from build123d import *

# Parameters (mm, degrees)
SKETCH1_R            = 28.1
SKETCH1_R_2          = 21.1
BOSS_EXTRUDE1_DEPTH  = 4.5
SKETCH2_R            = 28.1
SKETCH2_R_2          = 18.6
BOSS_EXTRUDE2_DEPTH  = 3
M3_CLEARANCE_HOLE1_D = 3.2
SKETCH6_R            = 3
CUT_EXTRUDE1_DEPTH   = 2
BOSS_EXTRUDE3_DEPTH  = 10
SKETCH8_R            = 2.125
CUT_EXTRUDE2_DEPTH   = 15
SKETCH9_W            = 6.5
SKETCH9_H            = 10
CUT_EXTRUDE3_DEPTH   = 7
CIRPATTERN1_COUNT    = 6
CIRPATTERN2_COUNT    = 2


with BuildPart() as part:
    # Sketch1 → Boss-Extrude1 (new body)
    with BuildSketch(Plane.XY):
        Circle(SKETCH1_R)
        Circle(SKETCH1_R_2, mode=Mode.SUBTRACT)
    extrude(amount=BOSS_EXTRUDE1_DEPTH)

    # Sketch2 → Boss-Extrude2 (add)
    with BuildSketch(Plane.XY.offset(4.5)):
        Circle(SKETCH2_R)
        Circle(SKETCH2_R_2, mode=Mode.SUBTRACT)
    extrude(amount=BOSS_EXTRUDE2_DEPTH)

    # M3 Clearance Hole1 (through all)
    with Locations(Plane(origin=(0, 0, 0), x_dir=(-1, 0, 0), z_dir=(0, 0, -1))):
        with Locations((0, 24.6)):
            m3_clearance_hole1 = Hole(M3_CLEARANCE_HOLE1_D / 2)

    # Sketch6 → Cut-Extrude1 (cut)
    with BuildSketch(Plane.XY.offset(7.5)):
        with Locations((0, 24.6)):
            Circle(SKETCH6_R)
    cut_extrude1 = extrude(amount=-CUT_EXTRUDE1_DEPTH, mode=Mode.SUBTRACT)

    # Sketch7 → Boss-Extrude3 (add)
    with BuildSketch(Plane.XY.offset(7.5)):
        Polygon((-6.504809472, 26.266660498), (-19.495190528, 18.766660498), (-15.995190528, 12.704482672), (-3.004809472, 20.204482672), align=None)
    boss_extrude3 = extrude(amount=BOSS_EXTRUDE3_DEPTH)

    # Sketch8 → Cut-Extrude2 (cut)
    with BuildSketch(Plane(origin=(-6.495190528, -3.75, 0), x_dir=(0, 0, 1), z_dir=(-0.866025404, -0.5, 0))):
        with Locations((14, 22.5)):
            Circle(SKETCH8_R)
    cut_extrude2 = extrude(amount=-CUT_EXTRUDE2_DEPTH, mode=Mode.SUBTRACT)

    # Sketch9 → Cut-Extrude3 (cut)
    with BuildSketch(Plane(origin=(-13, 22.516660498, 0), x_dir=(0.866025404, 0.5, 0), z_dir=(-0.5, 0.866025404, 0))):
        with Locations((0, -12.5)):
            Rectangle(SKETCH9_W, SKETCH9_H)
    cut_extrude3 = extrude(amount=-CUT_EXTRUDE3_DEPTH, mode=Mode.SUBTRACT)

    # CirPattern1: M3 Clearance Hole1, Cut-Extrude1 ×6 about axis
    cirpattern1_axis = Axis((0, 0, 0), (0, 0, 1))
    for i in range(1, CIRPATTERN1_COUNT):
        add(m3_clearance_hole1.rotate(cirpattern1_axis, i * 360 / CIRPATTERN1_COUNT), mode=Mode.SUBTRACT)
        add(cut_extrude1.rotate(cirpattern1_axis, i * 360 / CIRPATTERN1_COUNT), mode=Mode.SUBTRACT)

    # CirPattern2: Boss-Extrude3, Cut-Extrude2, Cut-Extrude3 ×2 about axis
    cirpattern2_axis = Axis((0, 0, 0), (0, 0, 1))
    for i in range(1, CIRPATTERN2_COUNT):
        add(boss_extrude3.rotate(cirpattern2_axis, i * 360 / CIRPATTERN2_COUNT))
        add(cut_extrude2.rotate(cirpattern2_axis, i * 360 / CIRPATTERN2_COUNT), mode=Mode.SUBTRACT)
        add(cut_extrude3.rotate(cirpattern2_axis, i * 360 / CIRPATTERN2_COUNT), mode=Mode.SUBTRACT)


solid = part.part
Can you work these out from the model? Positions are in its coordinate system, mm. A direction names the side the tool comes from. Give positions to 0.01 mm unless a question says otherwise; leave off trailing zeros. Write each loop counter-clockwise with the first axis right and the second up, starting at its lowest first coordinate (ties: lowest second). Pieces come first, ordered by that corner, then holes. Notation, with made-up numbers: M 5,44.25 L 38,44.25 A14 ccw 38,52.25 Z; hole C 62.25,-19.75 d3. An arc over 180 degrees is marked long. Answer in a Markdown table with one row per item. Add a question column.
Item 1: On a 3-axis mill with a long thin cutter (end or side, diameter ignored), from which of +Z, -Z, +X, -X, +Y, -Y can I reach the whole of each face in a straight line? I mean faces 5 (the cylindrical face through (-0.65, 21.67, 6.51)), 6 (the flat face through (17.77, -15.78, 11.32)), 7 (the flat face through (4.73, -23.19, 11.32)), 8 (the flat face through (14.089, -17.903, 11.459)). Say none if no direction works.
Item 2: For pin 1 Ø2 at (x, z) = (7, 9.5) entering from +Y; pin 2 Ø6.5 at (x, y) = (0, 26) entering from +Z; pin 3 Ø8 at (x, z) = (-18, 6) entering from -Y, each with a flat end and sliding along its axis, tell me the tip position at first contact or that it passes through.
Item 3: Imagine slicing it at B-B, the plane x = 0. Write out the boundary of the cut face in (y, z), plus the area to 3 significant figures.
Item 4: Imagine slicing it at D-D, the plane z = 15.25. State how many separate pieces and enclosed holes the cut face has, plus the area to 3 significant figures.
Item 5: We'd pull the mould along Y, two halves only. Please class faces 1 (the cylindrical face through (-6.092, -27.432, 3.698)), 2 (the cylindrical face through (6.668, -22.239, 11.877)), 3 (the flat face through (-17.629, 19.844, 12.43)), 4 (the flat face through (-17.77, 15.78, 11.32)): released by +Y, released by -Y, zero draft, split by the parting line, or undercut.
Item 6: Imagine slicing it at C-C, the plane y = 0. Write out the boundary of the cut face in (x, z).
Item 7: Imagine slicing it at A-A, the plane z = 9.5. Write out the boundary of the cut face in (x, y).
Item 8: Please list where these lines run through material, in increasing order: L1, parallel to Y at x = 0, z = 5.2; L2, parallel to Y at x = 0, z = 6.65; L3, parallel to Z at x = 17.5, y = 20.5.
Evaluation:
| question | item | result |
|---|---|---|
| 1 | face 5 | +Z |
| 1 | face 6 | +Z, +X, +Y |
| 1 | face 7 | +Z, -X, -Y |
| 1 | face 8 | +Z, -Y |
| 2 | pin 1 | stops at y = -18.08 |
| 2 | pin 2 | stops at z = 7.5 |
| 2 | pin 3 | stops at y = -24.36 |
| 3 | outline | M -28.1,0 L -26.2,0 L -26.2,5.5 L -27.6,5.5 L -27.6,7.5 L -28.1,7.5 Z; M -23,0 L -21.1,0 L -21.1,4.5 L -18.6,4.5 L -18.6,7.5 L -21.6,7.5 L -21.6,5.5 L -23,5.5 Z; M 18.6,4.5 L 21.1,4.5 L 21.1,0 L 23,0 L 23,5.5 L 21.6,5.5 L 21.6,7.5 L 18.6,7.5 Z; M 26.2,0 L 28.1,0 L 28.1,7.5 L 27.6,7.5 L 27.6,5.5 L 26.2,5.5 Z |
| 3 | area | 60.8 mm² |
| 4 | separate pieces | 8 |
| 4 | enclosed holes | 0 |
| 4 | area | 60.6 mm² |
| 5 | face 1 | split by the parting line |
| 5 | face 2 | undercut |
| 5 | face 3 | released by +Y |
| 5 | face 4 | released by -Y |
| 6 | outline | M -28.1,0 L -21.1,0 L -21.1,4.5 L -18.6,4.5 L -18.6,7.5 L -28.1,7.5 Z; M 18.6,4.5 L 21.1,4.5 L 21.1,0 L 28.1,0 L 28.1,7.5 L 18.6,7.5 Z |
| 7 | outline | M -19.5,18.77 L -16,12.7 L -12.31,14.83 L -15.81,20.89 Z; M -10.19,24.14 L -6.69,18.08 L -3,20.2 L -6.5,26.27 Z; M 3,-20.2 L 6.5,-26.27 L 10.19,-24.14 L 6.69,-18.08 Z; M 12.31,-14.83 L 15.81,-20.89 L 19.5,-18.77 L 16,-12.7 Z |
| 8 | L1 | y = -28.1 to -26.2, -23 to -18.6, 18.6 to 23, 26.2 to 28.1 |
| 8 | L2 | y = -28.1 to -27.6, -21.6 to -18.6, 18.6 to 21.6, 27.6 to 28.1 |
| 8 | L3 | z = 0 to 7.5 |
